Autodesk Inventor part; units mm, degrees
ref_plane "bolt_to_nut_XY" through (50, 0, 0) normal (1, 0, 0) x (0, 0, -1)
ref_plane "bolt_to_nut_YZ" through (50, 0, 0) normal (0, 0, -1) x (0, 1, 0)
ref_plane "bolt_to_nut_ZX" through (50, 0, 0) normal (0, 1, 0) x (1, 0, 0)
sketch "Sketch_2" plane through (0, 0, 0) normal (0, 0, 1) x (1, 0, 0)
  line L0 (50, 0) -> (-4, 0)
  line L1 (-4, 0) -> (-4, 3.1)
  line L2 (-4, 3.1) -> (-3.6, 3.5)
  line L3 (-3.6, 3.5) -> (0, 3.5)
  line L4 (0, 3.5) -> (0, 2)
  line L5 (0, 2) -> (49.5705, 2)
  line L6 (49.5705, 2) -> (50, 1.5705)
  line L7 (50, 1.5705) -> (50, 0)
  line L8 (50, 0) -> (-4, 0)
revolve "Revolution1" add sketch "Sketch_2" angle 360 about axis through (50, 0, 0) along (1, 0, 0)
thread "Thread1"
sketch "Sketch2" plane through (-4, 0, 0) normal (-1, 0, 0) x (0, 0, 1)
  point P0 (0, 0)
hole "Hole1" at (-4, 0, 0) direction (1, 0, 0) diameter 3 depth 2 tip angle 150
sketch "Sketch_3" plane through (-4, 0, 0) normal (1, 0, 0) x (0, 0, -1)
  line L0 (-1.5, -0.866) -> (0, -1.7321)
  line L1 (0, -1.7321) -> (1.5, -0.866)
  line L2 (1.5, -0.866) -> (1.5, 0.866)
  line L3 (1.5, 0.866) -> (0, 1.7321)
  line L4 (0, 1.7321) -> (-1.5, 0.866)
  line L5 (-1.5, 0.866) -> (-1.5, -0.866)
extrude "Extrusion1" cut sketch "Sketch_3" along normal blind 2
ref_plane "bolt_to_nut_XY" through (50, 0, 0) normal (1, 0, 0) x (0, 0, -1)
ref_plane "bolt_to_nut_YZ" through (50, 0, 0) normal (0, 0, -1) x (0, 1, 0)
ref_plane "bolt_to_nut_ZX" through (50, 0, 0) normal (0, 1, 0) x (1, 0, 0)
ref_plane "screw1_XY" through (0, 0, 0) normal (1, 0, 0) x (0, 0, -1)
ref_plane "screw1_YZ" through (0, 0, 0) normal (0, 0, -1) x (0, 1, 0)
ref_plane "screw1_ZX" through (0, 0, 0) normal (0, 1, 0) x (1, 0, 0)
properties part number "CB4-50" material "鋼、炭素鋼"
Source: CAD feature listing. Evaluate the final solid. Frame: model axes, mm. A direction names the side the tool comes from. Give positions to 0.01 mm unless a question says otherwise; leave off trailing zeros. Write each loop counter-clockwise with the first axis right and the second up, starting at its lowest first coordinate (ties: lowest second). Pieces come first, ordered by that corner, then holes.
1. First-contact query: pin 1 (4 mm diameter, centred on x = 35, y = 1.5, fed in from +Z); pin 2 (1.4 mm diameter, centred on x = -2.5, y = 0.5, fed in from +Z); pin 3 (1.5 mm diameter, centred on x = 39.5, z = -1.5, fed in from +Y); pin 4 (1 mm diameter, centred on x = 4.5, y = 1, fed in from +Z). Flat tips, straight axial feed; report the tip coordinate or a pass-through.
2. Access query for faces 1 (the face through (-3.014, -1.293, 0.76)), 2 (the face through (0, 2, -2)), 3 (the face through (-4, 1.3, -1.3)). Directions: +Z, -Z, +X, -X, +Y, -Y. A direction counts if a zero-diameter tool reaches every point of the face in a straight line with its end or side. Return the directions, or none.
3. Section query A-A (x = 41). Return the cut outline in (y, z).
4. Pull-direction query (Z, two-part tool) for faces 4 (the face through (50, 0, 0)), 5 (the face through (-1.775, 3.233, -1.341)), 6 (the face through (-3, 0, 1.5)); classes: +Z half, -Z half, draft (parallel to the pull), parting line (faces both ways), or undercut.
5. Material intervals for line 1 along Y through (x, z) = (16.5, -1); line 2 along X through (y, z) = (-1.5, -2); line 3 along Z through (x, y) = (18.5, -1.25), sorted ascending.
Output values:
1. pin 1: stops at z = 2
1. pin 2: stops at z = 3.5
1. pin 3: stops at y = 1.85
1. pin 4: stops at z = 1.94
2. face 1: -X
2. face 2: +X
2. face 3: +Z, -Z, -X, +Y, -Y
3. outline: circle Ø4 at (0, 0)
4. face 4: draft
4. face 5: parting line
4. face 6: undercut
5. line 1: y = -1.73 to 1.73
5. line 2: x = -4 to 0
5. line 3: z = -1.56 to 1.56
